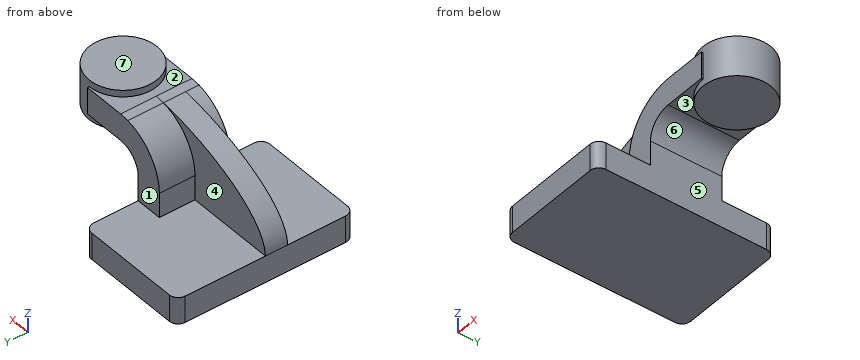
```python
from build123d import *

# Parameters (mm, degrees)
F1_DEPTH = 63.5
F0_W     = 26.7074994694
F0_H     = 19.05
F2_DEPTH = 25.4
F3_DEPTH = 15.875
F5_R     = 6.35


with BuildPart() as f1:
    # F0 (on Front) → F1 (new body, symmetric)
    with BuildSketch(Plane.XZ):
        Polygon((-41.275, -9.525), (41.275, -9.525), (41.275, 9.525), (22.225, 9.525), (-41.275, 9.525), align=None)
    extrude(amount=F1_DEPTH, both=True)

    # F0 (on Front) → F2 (join, symmetric)
    with BuildSketch(Plane.XZ):
        with BuildLine():
            Line((22.225, 9.525), (41.275, 9.525))
            Line((41.275, 9.525), (41.275, 27.0002))
            ThreePointArc((41.275, 27.0002), (45.9246798487, 38.2255201513), (57.15, 42.8752))
            Line((57.15, 42.8752), (60.325, 42.8752))
            Line((60.325, 42.8752), (60.325, 61.9252))
            Line((60.325, 61.9252), (57.15, 61.9252))
            add(Edge.make_bspline(
                [(50.7148259904, 61.3272179373), (52.8977826503, 61.5734874191), (55.0462400607, 61.7732473961), (57.15, 61.9252)],
                knots=[105.6945195788, 105.6945195788, 105.6945195788, 105.6945195788, 111.5045361635, 111.5045361635, 111.5045361635, 111.5045361635], degree=3))
            ThreePointArc((50.7148259904, 61.3272179373), (30.2752527706, 49.3049884177), (22.225, 27.0002))
            Line((22.225, 27.0002), (22.225, 9.525))
        make_face()
        with Locations((73.6787497347, 52.4002)):
            Rectangle(F0_W, F0_H)
    extrude(amount=F2_DEPTH, both=True)

    # F0 (on Front) → F3 (join)
    with BuildSketch(Plane.XZ):
        with BuildLine():
            add(Edge.make_bspline(
                [(-41.275, 9.525), (-40.1260967037, 36.9751709766), (11.0029676748, 56.8471387181), (50.7148259904, 61.3272179373)],
                knots=[0, 0, 0, 0, 105.6945195788, 105.6945195788, 105.6945195788, 105.6945195788], degree=3))
            Line((-41.275, 9.525), (22.225, 9.525))
            Line((22.225, 9.525), (22.225, 27.0002))
            ThreePointArc((22.225, 27.0002), (30.2752527706, 49.3049884177), (50.7148259904, 61.3272179373))
        make_face()
    extrude(amount=F3_DEPTH)

    # F0 (on Front) → F4 (revolve)
    with BuildSketch(Plane.XZ):
        Polygon((87.0324994694, 61.9252), (87.0324994694, 42.8752), (87.0324994694, 38.1), (111.125, 38.1), (111.125, 66.675), (87.0324994694, 66.675), align=None)
    revolve(axis=Axis((87.0324994694, 0, 52.3875), (0, 0, -1)))

    # F5
    f5_edges = [f1.edges().sort_by_distance(p)[0] for p in [
        (41.275, -63.5, 0),
        (-41.275, -63.5, 0),
        (41.275, 63.5, 0),
        (-41.275, 63.5, 0),
    ]]
    fillet(f5_edges, radius=F5_R)


solid = f1.part
```
Could you check a few things on this model? Use its own coordinates, in mm. Face numbers are marked on the shaded views. A direction names the side the tool comes from. Round coordinates to 2 decimals unless told otherwise and drop trailing zeros. Write each loop counter-clockwise with the first axis right and the second up, starting at its lowest first coordinate (ties: lowest second). Pieces come first, ordered by that corner, then holes. Notation, with made-up numbers: M 38,10.25 L 66,10.25 A28 ccw 66,34.25 Z; hole C 33,34.5 d9. An arc over 180 degrees is marked long. Write each question's results on one line, items separated by ' | '. Start each with the question number.
1. I need wall thicknesses on L1, parallel to Y at x = -1, z = 18 (3 decimals); L2, parallel to X at y = 42, z = 5.5 (3 decimals); L3, parallel to Z at x = 28.5, y = 36 (3 decimals). Which ranges of each line are inside material? Lowest first, please. Write a range as from..to.
2. Imagine slicing it at A-A on z = 7.5. List the corners of the cut face in (x, y) for me (3 decimals), and give its area (3 significant figures).
3. Imagine slicing it at B-B on y = -34. List the corners of the cut face in (x, z) for me (3 decimals), and give its area (3 significant figures).
4. I'm going to push flat-ended pins straight in: pin 1 Ø2 at (y, z) = (-3, 36) entering from +X; pin 2 Ø7.5 at (y, z) = (-21.5, 19) entering from -X (3 decimals); pin 3 Ø4 at (x, y) = (-9.5, -34.5) entering from +Z (3 decimals). Where does each tip first touch, or does it pass through?
5. Thinking about a two-plate mould opening in X: for the marked faces 5, 6 and 7, which applies, +X half, -X half, draft (parallel to the pull), parting line (faces both ways), or undercut?
6. On a 3-axis mill with a long thin cutter (end or side, diameter ignored), from which of +Z, -Z, +X, -X, +Y, -Y can I reach the whole of each face in a straight line? I mean the marked faces 1, 2, 3 and 4. Say none if no direction works.
Result sheet:
1) L1: y = -15.875..0 | L2: x = -41.275..41.275 | L3: z = -9.525..9.525
2) outline: M -41.275,-57.15 A6.35 ccw -34.925,-63.5 L 34.925,-63.5 A6.35 ccw 41.275,-57.15 L 41.275,57.15 A6.35 ccw 34.925,63.5 L -34.925,63.5 A6.35 ccw -41.275,57.15 Z | area: 10,400 mm^2
3) outline: M -41.275,-9.525 L 41.275,-9.525 L 41.275,9.525 L -41.275,9.525 Z | area: 1,570 mm^2
4) pin 1: stops at x = 44.82 | pin 2: stops at x = 22.225 | pin 3: stops at z = 9.525
5) face 5: +X half | face 6: undercut | face 7: draft
6) face 1: +Z, +X, -X, +Y | face 2: +Z, -X | face 3: -Z | face 4: +Z, -X, +Y
